```python
from build123d import *

# Parameters (mm, degrees)
F0_R      = 1.59
F1_DEPTH  = 5
F2_W      = 74.4103554785
F2_H      = 125.3275879622
F3_DEPTH  = 32
F4_R      = 2.7900010005
F4_R_2    = 2.7899997517
F4_R_3    = 2.79
F5_DEPTH  = 2
F6_DEPTH  = 37.001
F8_DEPTH  = 2.6
F9_W      = 13
F9_H      = 12.5
F9_W_2    = 10.5
F9_H_2    = 14.01349
F9_W_3    = 6.5
F9_H_3    = 4
F10_DEPTH = 3
F9_W_4    = 17.9999999672
F9_H_4    = 10.5999999672
F9_W_5    = 14.8
F9_H_5    = 7.4
F11_DEPTH = 7
F13_DEPTH = 6
F14_R     = 1
F15_DEPTH = 125.3285879622
F16_R     = 1.5
F17_DEPTH = 3


# Not quite as in the source:
# - a feature names something its author has since deleted; it is built from what else it names


with BuildPart() as f1:
    # F0 (on Top) → F1 (new body)
    with BuildSketch(Plane.XY):
        Polygon((27.9103554785, 29), (-46.5, 29), (-46.5, -29), (-46.5, -96.3275879622), (27.9103554785, -96.3275879622), align=None)
        with Locations((-30.1368717179, -24.2969288903)):
            Circle(F0_R, mode=Mode.SUBTRACT)
        with Locations((-28.8368717179, 24.0430711097)):
            Circle(F0_R, mode=Mode.SUBTRACT)
        with Locations((21.9631282821, -19.0569288903)):
            Circle(F0_R, mode=Mode.SUBTRACT)
        with Locations((21.9631282821, 8.8430711097)):
            Circle(F0_R, mode=Mode.SUBTRACT)
        with Locations((21.9631282821, -19.0569288903)):
            Circle(F0_R)
        with Locations((-28.8368717179, 24.0430711097)):
            Circle(F0_R)
        with Locations((-30.1368717179, -24.2969288903)):
            Circle(F0_R)
        with Locations((21.9631282821, 8.8430711097)):
            Circle(F0_R)
    extrude(amount=F1_DEPTH)

    # F2 (on face) → F3 (join)
    with BuildSketch(Plane.XY.offset(5)):
        with Locations((-9.2948222607, -33.6637939811)):
            Rectangle(F2_W, F2_H)
        Polygon((25.9103551507, 26.9999996722), (25.9103551507, -94.3275876343), (-44.4999996722, -94.3275876343), (-44.4999996722, -29), (-44.4999996722, 26.9999996722), align=None, mode=Mode.SUBTRACT)
    extrude(amount=F3_DEPTH)

    # F4 (on face) → F5 (join)
    with BuildSketch(Plane.XY.offset(5)):
        with Locations((-28.8368717179, 24.0430711097)):
            Circle(F4_R)
        with Locations((21.9631282821, 8.8430711097)):
            Circle(F4_R_2)
        with Locations((21.9631282821, -19.0569288903)):
            Circle(F4_R_3)
        with Locations((-30.1368717179, -24.2969288903)):
            Circle(F4_R_3)
    extrude(amount=F5_DEPTH)

    # F0 (on Top) → F6 (cut, through all)
    with BuildSketch(Plane.XY):
        with Locations((-30.1368717179, -24.2969288903)):
            Circle(F0_R)
        with Locations((21.9631282821, -19.0569288903)):
            Circle(F0_R)
        with Locations((21.9631282821, 8.8430711097)):
            Circle(F0_R)
        with Locations((-28.8368717179, 24.0430711097)):
            Circle(F0_R)
    extrude(amount=F6_DEPTH, mode=Mode.SUBTRACT)

    # F7 (on Top) → F8 (cut)
    with BuildSketch(Plane.XY):
        Polygon((-28.5388533662, -27.1075641711), (-26.9037809882, -24.3183220425), (-28.5017993398, -21.5076867618), (-31.7348900695, -21.4862936096), (-33.3699624476, -24.2755357382), (-31.7719440959, -27.0861710189), align=None)
        Polygon((23.649281557, -21.8155916945), (25.1952769884, -18.9760087217), (23.5091237135, -16.2173459175), (20.2769750072, -16.2982660862), (18.7309795758, -19.137849059), (20.4171328507, -21.8965118631), align=None)
        Polygon((23.5751015985, 6.040416054), (25.1962854165, 8.837753424), (23.5843121002, 11.6404084796), (20.3511549658, 11.6457261653), (18.7299711478, 8.8483887953), (20.3419444641, 6.0457337397), align=None)
        Polygon((-28.8368717179, 20.8099096022), (-26.0368717179, 22.4264903559), (-26.0368717179, 25.6596518634), (-28.8368717179, 27.2762326171), (-31.6368717179, 25.6596518634), (-31.6368717179, 22.4264903559), align=None)
    extrude(amount=F8_DEPTH, mode=Mode.SUBTRACT)

    # F9 (on face) → F10 (cut)
    with BuildSketch(Plane(origin=(-46.5, 0, 0), x_dir=(0, -1, 0), z_dir=(-1, 0, 0))):
        with Locations((-11.010112679, 13.25)):
            Rectangle(F9_W, F9_H)
        with Locations((18.2770747468, 14.006745)):
            Rectangle(F9_W_2, F9_H_2)
        with Locations((-14.260112679, 25.6000000164)):
            Rectangle(F9_W_3, F9_H_3)
    extrude(amount=-F10_DEPTH, mode=Mode.SUBTRACT)

    # F9 (on face) → F11 (join)
    with BuildSketch(Plane(origin=(-46.5, 0, 0), x_dir=(0, -1, 0), z_dir=(-1, 0, 0))):
        with Locations((-14.260112679, 25.6000000164)):
            Rectangle(F9_W_4, F9_H_4)
        with Locations((-14.260112679, 25.6000000164)):
            Rectangle(F9_W_5, F9_H_5, mode=Mode.SUBTRACT)
    extrude(amount=-F11_DEPTH)

    # F12 (on face) → F13 (cut)
    with BuildSketch(Plane.XY.offset(5)):
        with BuildLine():
            ThreePointArc((-40.7473873347, 2.5), (-41.9973873347, 1.25), (-40.7473873347, 0))
            Line((-40.7473873347, 0), (-10.7473873347, 0))
            ThreePointArc((-10.7473873347, 0), (-9.4973873347, 1.25), (-10.7473873347, 2.5))
            Line((-10.7473873347, 2.5), (-40.7473873347, 2.5))
        make_face()
        with BuildLine():
            ThreePointArc((-40.7473873347, -2.0948293991), (-41.9973873347, -3.3448293991), (-40.7473873347, -4.5948293991))
            Line((-40.7473873347, -4.5948293991), (-10.7473873347, -4.5948293991))
            ThreePointArc((-10.7473873347, -4.5948293991), (-9.4973873347, -3.3448293991), (-10.7473873347, -2.0948293991))
            Line((-10.7473873347, -2.0948293991), (-40.7473873347, -2.0948293991))
        make_face()
        with BuildLine():
            ThreePointArc((-40.7473873347, -6.6774361208), (-41.9973873347, -7.9274361208), (-40.7473873347, -9.1774361208))
            Line((-40.7473873347, -9.1774361208), (-10.7473873347, -9.1774361208))
            ThreePointArc((-10.7473873347, -9.1774361208), (-9.4973873347, -7.9274361208), (-10.7473873347, -6.6774361208))
            Line((-10.7473873347, -6.6774361208), (-40.7473873347, -6.6774361208))
        make_face()
        with BuildLine():
            ThreePointArc((-40.7473873347, -11.2855438516), (-41.9973873347, -12.5355438516), (-40.7473873347, -13.7855438516))
            Line((-40.7473873347, -13.7855438516), (-10.7473873347, -13.7855438516))
            ThreePointArc((-10.7473873347, -13.7855438516), (-9.4973873347, -12.5355438516), (-10.7473873347, -11.2855438516))
            Line((-10.7473873347, -11.2855438516), (-40.7473873347, -11.2855438516))
        make_face()
        with BuildLine():
            ThreePointArc((-40.7473873347, -15.9455886483), (-41.9973873347, -17.1955886483), (-40.7473873347, -18.4455886483))
            Line((-40.7473873347, -18.4455886483), (-10.7473873347, -18.4455886483))
            ThreePointArc((-10.7473873347, -18.4455886483), (-9.4973873347, -17.1955886483), (-10.7473873347, -15.9455886483))
            Line((-10.7473873347, -15.9455886483), (-40.7473873347, -15.9455886483))
        make_face()
        with BuildLine():
            ThreePointArc((-40.7473873347, 6.6440958157), (-41.9973873347, 5.3940958157), (-40.7473873347, 4.1440958157))
            Line((-40.7473873347, 4.1440958157), (-10.7473873347, 4.1440958157))
            ThreePointArc((-10.7473873347, 4.1440958157), (-9.4973873347, 5.3940958157), (-10.7473873347, 6.6440958157))
            Line((-10.7473873347, 6.6440958157), (-40.7473873347, 6.6440958157))
        make_face()
        with BuildLine():
            ThreePointArc((-40.7473873347, 11.013558656), (-41.9973873347, 9.763558656), (-40.7473873347, 8.513558656))
            Line((-40.7473873347, 8.513558656), (-10.7473873347, 8.513558656))
            ThreePointArc((-10.7473873347, 8.513558656), (-9.4973873347, 9.763558656), (-10.7473873347, 11.013558656))
            Line((-10.7473873347, 11.013558656), (-40.7473873347, 11.013558656))
        make_face()
        with BuildLine():
            ThreePointArc((-40.7473873347, 15.4895936698), (-41.9973873347, 14.2395936698), (-40.7473873347, 12.9895936698))
            Line((-40.7473873347, 12.9895936698), (-10.7473873347, 12.9895936698))
            ThreePointArc((-10.7473873347, 12.9895936698), (-9.4973873347, 14.2395936698), (-10.7473873347, 15.4895936698))
            Line((-10.7473873347, 15.4895936698), (-40.7473873347, 15.4895936698))
        make_face()
        with BuildLine():
            ThreePointArc((-40.7473873347, 19.7524824739), (-41.9973873347, 18.5024824739), (-40.7473873347, 17.2524824739))
            Line((-40.7473873347, 17.2524824739), (-10.7473873347, 17.2524824739))
            ThreePointArc((-10.7473873347, 17.2524824739), (-9.4973873347, 18.5024824739), (-10.7473873347, 19.7524824739))
            Line((-10.7473873347, 19.7524824739), (-40.7473873347, 19.7524824739))
        make_face()
    extrude(amount=F13_DEPTH, mode=Mode.SUBTRACT)

    # F14 (on face) → F15 (cut, through all)
    with BuildSketch(Plane.XZ.offset(96.3275879622)):
        with Locations((-9.2948222607, 34)):
            Circle(F14_R)
    extrude(amount=-F15_DEPTH, mode=Mode.SUBTRACT)

    # F16 (on face) → F17 (cut)
    with BuildSketch(Plane.YZ.offset(27.9103554785)):
        with Locations((-27.9986988753, 7.8254723921)):
            Circle(F16_R)
    extrude(amount=-F17_DEPTH, mode=Mode.SUBTRACT)


solid = f1.part
```
The model under review builds one solid part; all positions refer to its coordinate system, in mm. A direction names the side the tool comes from. Round coordinates to 2 decimals unless told otherwise and drop trailing zeros. Write each loop counter-clockwise with the first axis right and the second up, starting at its lowest first coordinate (ties: lowest second). Pieces come first, ordered by that corner, then holes. Notation, with made-up numbers: (37, 49.25) - (85, 49.25) arc R27 cw to (85, 85.25) - close; hole circle Ø11 at (89, 81.5). An arc over 180 degrees is marked (long way). Use one line per item in the form item = value.
Q1. For line 1 (Y direction, x = 18, z = 21.5); line 2 (X direction, y = -83.5, z = 10); line 3 (Y direction, x = -30.5, z = 2), list the stretches that pass through material, from the lowest coordinate up. Write a range as [from, to].
Answer key:
line_1 = [-96.33, -94.33], [27, 29]
line_2 = [-46.5, -44.5], [25.91, 27.91]
line_3 = [-96.33, -27.09], [-21.49, 21.77], [26.32, 29]
Q2. Consider section A-A (x = 6). State the section outline as (y, z) points, and give its area (3 significant figures).
Answer key:
outline = (-96.33, 0) - (29, 0) - (29, 37) - (27, 37) - (27, 5) - (-94.33, 5) - (-94.33, 37) - (-96.33, 37) - close
area = 755 mm2
Q3. Draft analysis for pull direction Z (two halves, no side actions). For faces 1 (the flat face through (23.2, -20.3, 7)), 2 (the cylindrical face through (26.924, -29.497, 7.891)), 3 (the flat face through (27.91, -35, 18)), state which applies: +Z half, -Z half, draft (parallel to the pull), parting line (faces both ways), or undercut.
Answer key:
face_1 = +Z half
face_2 = undercut
face_3 = draft
Q4. Consider section B-B (y = -34.5). State the section outline as (x, z) points.
Answer key:
outline = (-46.5, 0) - (27.91, 0) - (27.91, 37) - (25.91, 37) - (25.91, 5) - (-44.5, 5) - (-44.5, 37) - (-46.5, 37) - close
Q5. Tool access review of faces 4 (the cylindrical face through (-29.403, -25.708, 4.769)), 5 (the flat face through (24.41, -20.42, 1.28)), 6 (the flat face through (25.91, -33, 21)): name each direction out of +Z, -Z, +X, -X, +Y, -Y from which nothing blocks a thin tool from reaching the whole face with its end or side.
Answer key:
face_4 = +Z, -Z
face_5 = -Z
face_6 = +Z
Q6. Insertion check: pin 1 Ø3 at (x, y) = (13.5, -73.5) entering from +Z; pin 2 Ø6 at (y, z) = (-19, 10.5) entering from -X; pin 3 Ø1.7 at (x, y) = (-29, -23.5) entering from +Z. Each pin has a flat end and moves straight along its axis. Give the tip position at first contact, or say it passes through.
Answer key:
pin_1 = 5
pin_2 = 25.91
pin_3 = 7
